```python
from build123d import *

# Parameters (mm, degrees)
F0_W      = 9.652
F0_H      = 16.9672
F1_DEPTH  = 12.192
F2_DEPTH  = 2.9972
F4_DEPTH  = 25.4
F6_DEPTH  = 3.2385
F8_DEPTH  = 3.2385
F10_D     = 6.7564
F10_DEPTH = 15.7734
F10_TIP   = 2.0298273432


with BuildPart() as f1:
    # F0 (on Front) → F1 (new body)
    with BuildSketch(Plane.XZ):
        with Locations((0, 26.8224)):
            Rectangle(F0_W, F0_H)
        with BuildLine():
            Line((4.826, 18.3388), (-4.826, 18.3388))
            Line((-4.826, 18.3388), (-8.0645, 18.3388))
            Line((-8.0645, 18.3388), (-8.0645, 4.826))
            ThreePointArc((-8.0645, 4.826), (0, 6.731), (8.0645, 4.826))
            Line((8.0645, 4.826), (8.0645, 18.3388))
            Line((8.0645, 18.3388), (4.826, 18.3388))
        make_face()
        with BuildLine():
            ThreePointArc((8.0645, 4.826), (0, 6.731), (-8.0645, 4.826))
            Line((-8.0645, 4.826), (-8.0645, 0))
            Line((-8.0645, 0), (8.0645, 0))
            Line((8.0645, 0), (8.0645, 4.826))
        make_face()
    extrude(amount=F1_DEPTH)

    # F0 (on Front) → F2 (join)
    with BuildSketch(Plane.XZ):
        with BuildLine():
            ThreePointArc((8.0645, 4.826), (0, 6.731), (-8.0645, 4.826))
            Line((-8.0645, 4.826), (-8.0645, 0))
            Line((-8.0645, 0), (8.0645, 0))
            Line((8.0645, 0), (8.0645, 4.826))
        make_face()
    extrude(amount=-F2_DEPTH)

    # F3 (on face) → F4 (cut, symmetric)
    with BuildSketch(Plane(origin=(-4.826, 0, 0), x_dir=(0, -1, 0), z_dir=(-1, 0, 0))):
        Polygon((2.159, 37.6501940191), (2.159, 35.306), (9.652, 26.924), (9.652, 17.5997419355), (12.192, 16.256), (15.097416006, 16.256), (15.097416006, 26.924), (15.097416006, 37.6501940191), align=None)
    extrude(amount=F4_DEPTH, both=True, mode=Mode.SUBTRACT)

    # F5 (on face) → F6 (cut, through all)
    with BuildSketch(Plane(origin=(-4.826, 0, 0), x_dir=(0, -1, 0), z_dir=(-1, 0, 0))):
        Polygon((9.652, 17.5997419355), (9.652, 18.3388), (8.255, 18.3388), align=None)
    extrude(amount=F6_DEPTH, mode=Mode.SUBTRACT)

    # F7 (on face) → F8 (cut, through all)
    with BuildSketch(Plane.YZ.offset(4.826)):
        Polygon((-8.255, 18.3388), (-9.652, 18.3388), (-9.652, 17.5997419355), align=None)
    extrude(amount=F8_DEPTH, mode=Mode.SUBTRACT)

    # F10
    with Locations(Plane(origin=(0, 0, 0), x_dir=(1, 0, 0), z_dir=(0, 0, -1))):
        with Locations((0, 5.588)):
            Hole(F10_D / 2, depth=F10_DEPTH)
            with Locations((0, 0, -(F10_DEPTH + F10_TIP / 2))):  # 118° drill point
                Cone(0, F10_D / 2, F10_TIP, mode=Mode.SUBTRACT)


solid = f1.part
```
Input: part model. Units: mm. Frame: model coordinates. A direction names the side the tool comes from. Give positions to 0.01 mm unless a question says otherwise; leave off trailing zeros. Write each loop counter-clockwise with the first axis right and the second up, starting at its lowest first coordinate (ties: lowest second). Pieces come first, ordered by that corner, then holes. Notation, with made-up numbers: (77.5, 50) - (86.5, 50) arc R25 ccw to (86.5, 73) - close; hole circle Ø11 at (70, 25). An arc over 180 degrees is marked (long way). Write item = value, one per line. Start each with the question number.
1) Cut plane A-A (y = 0.5). Return loops of the section in (x, z), and give its area (3 significant figures).
2) Material intervals for L1, parallel to Y at x = 0, z = 10.75; L2, parallel to X at y = -4.25, z = 6; L3, parallel to Y at x = 4, z = 16, sorted ascending. Write a range as [from, to].
3) Reachability of faces 1 (the face through (0, -1, 35.306)), 2 (the face through (0, -9.652, 22)), 3 (the face through (6, -4, 18.339)) from +Z, -Z, +X, -X, +Y, -Y: full face, straight path, thin tool, end or side. Return the list, or none.
4) Cut plane C-C (x = 5.5). Return loops of the section in (y, z) (3 decimals).
5) Cut plane D-D (z = 29). Return loops of the section in (x, y).
6) Pin query (flat end, axial travel): pin 1 (3.5 mm diameter, centred on x = 7, y = -2.5, fed in from +Z); pin 2 (3 mm diameter, centred on y = -2.5, z = 24, fed in from -X); pin 3 (2 mm diameter, centred on y = -10.5, z = 23, fed in from +X); pin 4 (5 mm diameter, centred on x = 1, y = -10.5, fed in from -Z). Return the tip coordinate at first contact, or that it passes through.
7) Cut plane B-B (z = 10.5). Return loops of the section in (x, y), and give its area (3 significant figures).
8) Draft query along X for faces 4 (the face through (-1.816, -8.437, 7.997)), 5 (the face through (-6, -4, 18.339)), 6 (the face through (0.12, 1.48, 6.73)). Return one class per face: pulls with the +X half, pulls with the -X half, needs draft (parallel to the pull), parting line crosses it, or undercut.
Answers follow:
q1.outline = (-8.06, 0) - (8.06, 0) - (8.06, 4.83) arc R18.02 ccw to (-8.06, 4.83) - close
q1.area = 98.5 mm^2
q2.L1 = [-12.19, -8.97], [-2.21, 0]
q2.L2 = [-8.06, -3.1], [3.1, 8.06]
q2.L3 = [-12.19, 0]
q3.face_1 = +Z, +X, -X, +Y, -Y
q3.face_2 = +Z, +X, -X, -Y
q3.face_3 = +Z, +X, +Y, -Y
q4.outline = (-12.192, 0) - (2.997, 0) - (2.997, 5.871) - (0, 5.871) - (0, 18.339) - (-8.255, 18.339) - (-12.192, 16.256) - close
q5.outline = (-4.83, -7.8) - (4.83, -7.8) - (4.83, 0) - (-4.83, 0) - close
q6.pin_1 = 18.34
q6.pin_2 = -4.83
q6.pin_3 = 4.83
q6.pin_4 = 0
q7.outline = (-8.06, -12.19) - (8.06, -12.19) - (8.06, 0) - (-8.06, 0) - close; hole circle Ø6.76 at (0, -5.59)
q7.area = 161 mm^2
q8.face_4 = undercut
q8.face_5 = needs draft
q8.face_6 = parting line crosses it
